Source: CAD feature listing. Evaluate the final solid. Frame: model axes, mm. Face numbers are marked on the shaded views. Round coordinates to 2 decimals unless told otherwise and drop trailing zeros. Order: outer loops, then holes, each group sorted by start corner. A loop starts at its lowest first (then second) coordinate and runs counter-clockwise, first axis right, second up. Notation, with made-up numbers: M 75.25,23 L 91.25,23 A12 cw 91.25,31 Z; hole C 45.25,20.25 d6. An arc over 180 degrees is marked long. Answer in a Markdown table with one row per item. Add a question column.
```python
from build123d import *

# Parameters (mm, degrees)
SKETCH1_W           = 248.6
SKETCH1_H           = 179.5
BOSS_EXTRUDE1_DEPTH = 20
SKETCH2_W           = 242.6
SKETCH2_H           = 173.5
CUT_EXTRUDE1_DEPTH  = 0.25
SKETCH3_W           = 5
SKETCH3_H           = 5
BOSS_EXTRUDE2_DEPTH = 0.75
SKETCH4_R           = 2.75
CUT_EXTRUDE2_DEPTH  = 9
SKETCH6_R           = 1.05
BOSS_EXTRUDE3_DEPTH = 6
FILLET1_R           = 0.25


with BuildPart() as part:
    # Sketch1 → Boss-Extrude1 (new body)
    with BuildSketch(Plane.XY):
        Rectangle(SKETCH1_W, SKETCH1_H)
    extrude(amount=BOSS_EXTRUDE1_DEPTH)

    # Sketch2 → Cut-Extrude1 (cut)
    with BuildSketch(Plane.XY.offset(20)):
        Rectangle(SKETCH2_W, SKETCH2_H)
    extrude(amount=-CUT_EXTRUDE1_DEPTH, mode=Mode.SUBTRACT)

    # Sketch3 → Boss-Extrude2 (add)
    with BuildSketch(Plane(origin=(124.3, 0, 0), x_dir=(0, 0, -1), z_dir=(1, 0, 0))):
        with Locations((-10, 69.75)):
            Rectangle(SKETCH3_W, SKETCH3_H)
        with Locations((-10, 0)):
            Rectangle(SKETCH3_W, SKETCH3_H)
        with Locations((-10, -69.75)):
            Rectangle(SKETCH3_W, SKETCH3_H)
    extrude(amount=BOSS_EXTRUDE2_DEPTH)

    # Sketch4 → Cut-Extrude2 (cut)
    with BuildSketch(Plane.ZY.offset(124.3)):
        with Locations(Location((10, 81.631746132, 0), (0, 0, 270))):
            Circle(SKETCH4_R)
    extrude(amount=-CUT_EXTRUDE2_DEPTH, mode=Mode.SUBTRACT)

    # Sketch6 → Boss-Extrude3 (add)
    with BuildSketch(Plane.ZY.offset(115.3)):
        with Locations(Location((10, 81.631746132, 0), (0, 0, 270))):
            Circle(SKETCH6_R)
    extrude(amount=BOSS_EXTRUDE3_DEPTH)

    # Fillet1
    fillet1_edges = [part.edges().sort_by_distance(p)[0] for p in [
        (-121.3, 82.681746132, 10),
    ]]
    fillet(fillet1_edges, radius=FILLET1_R)


solid = part.part
```
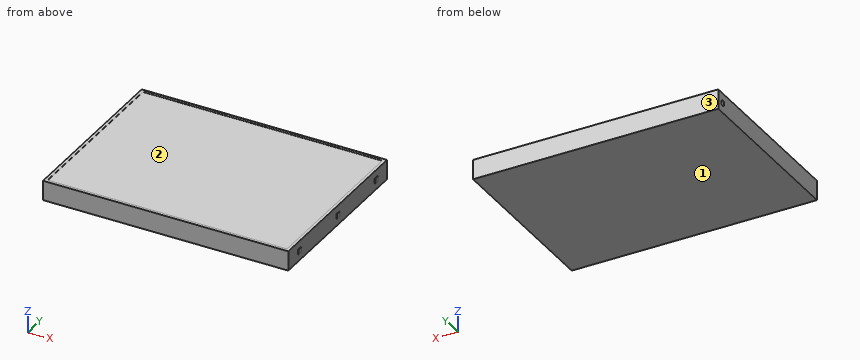
(1) Pin query (flat end, axial travel): pin 1 (0.8 mm diameter, centred on x = 125, y = -70, fed in from +Z); pin 2 (8 mm diameter, centred on y = -56, z = 2.5, fed in from +X); pin 3 (6 mm diameter, centred on x = -54, y = -58, fed in from +Z). Return the tip coordinate at first contact, or that it passes through.
(2) Cut plane A-A (y = 44). Return loops of the section in (x, z).
(3) Line query: line 1 (X direction, y = 62, z = 9.25); line 2 (Z direction, x = -9, y = -40.5). Output: solid intervals per line, ascending. Write a range as from..to.
(4) Draft query along Y for the marked faces 1, 2 and 3. Return one class per face: +Y half, -Y half, draft (parallel to the pull), parting line (faces both ways), or undercut.
Answer list:
| question | item | result |
|---|---|---|
| 1 | pin 1 | z = 12.5 |
| 1 | pin 2 | x = 124.3 |
| 1 | pin 3 | z = 19.75 |
| 2 | outline | M -124.3,0 L 124.3,0 L 124.3,20 L 121.3,20 L 121.3,19.75 L -121.3,19.75 L -121.3,20 L -124.3,20 Z |
| 3 | line 1 | -124.3..124.3 |
| 3 | line 2 | 0..19.75 |
| 4 | face 1 | draft |
| 4 | face 2 | undercut |
| 4 | face 3 | +Y half |
